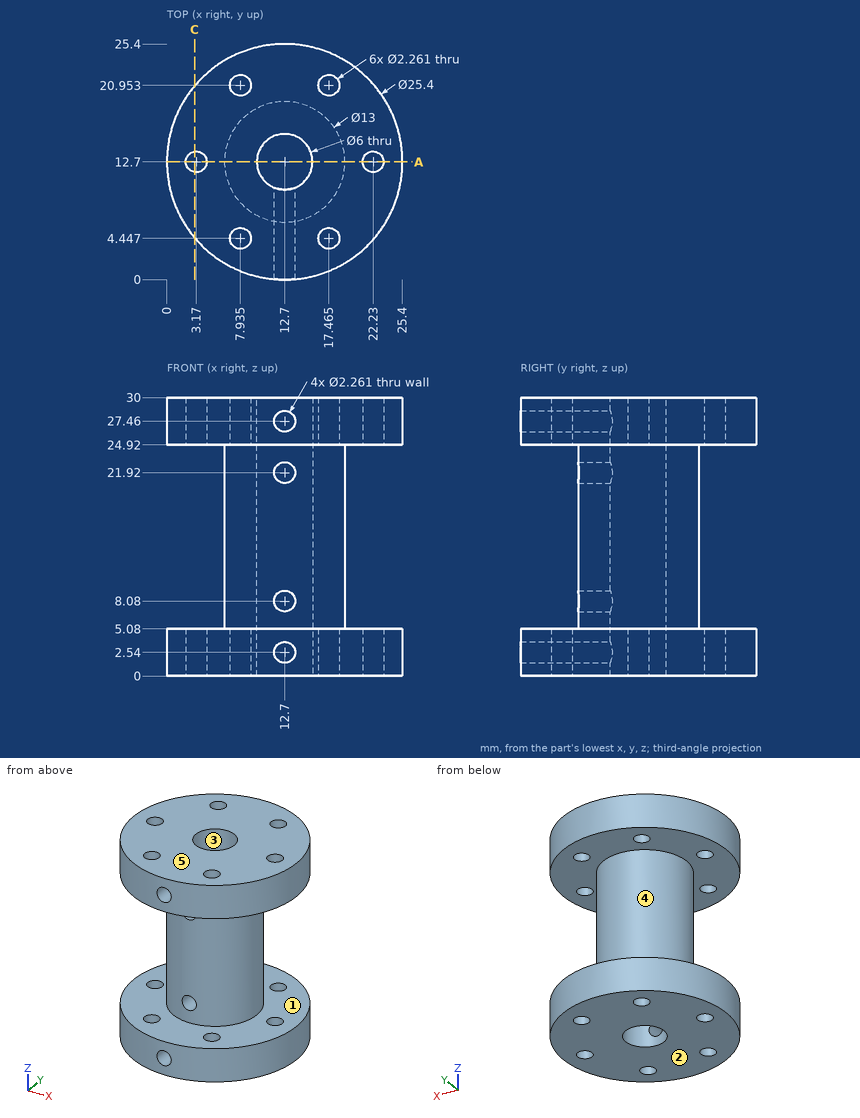
The figure shows three views and two pictorial views of one solid part (mm, origin at its lowest corner). Answer the questions. A direction names the side the tool comes from. Round coordinates to 2 decimals unless told otherwise and drop trailing zeros. Loops run counter-clockwise (first coordinate to the right, second up) from the corner with the lowest first, then second, coordinate; pieces in that order, holes last. Notation, with made-up numbers: (-23, 28) - (11, 28) arc R15 cw to (11, 43) - close; hole circle Ø2 at (32.25, -8.5). An arc over 180 degrees is marked (long way). One line per question, with ' | ' between items. Start each with the question number.
Q1. Flat-ended cylindrical pins translate along their axes: pin 1 (10 mm diameter, centred on x = 19.5, z = 17.5, fed in from -Y); pin 2 (6 mm diameter, centred on x = 9, z = 18, fed in from -Y); pin 3 (5 mm diameter, centred on x = 20, z = 13.5, fed in from -Y). Find the tip coordinate at first contact, or state that the pin passes through.
Q2. Section A-A on y = 12.7 is taken. Count the separate pieces of the cut face and the enclosed holes in it, plus the area to 3 significant figures.
Q3. Section C-C on x = 3 is taken. Give the vertices of the cut face in (y, z), plus the area to 3 significant figures.
Q4. For a pull along X with two mould halves and no side action, classify the marked faces 3, 4 and 5 as +X half, -X half, draft (parallel to the pull), parting line (faces both ways), or undercut.
Q5. For the marked faces 1 and 2, determine the directions among +Z, -Z, +X, -X, +Y, -Y from which every point of the face is accessible in a straight line to the end or side of a thin tool.
Q6. Find the intervals of material crossed by L1, parallel to Z at x = 12.7, y = 7.6; L2, parallel to Z at x = 20.5, y = 12.25; L3, parallel to Y at x = 12.7, z = 7, in increasing order.
Established:
1) pin 1: y = 6.45 | pin 2: y = 6.24 | pin 3: y = 8.32
2) separate pieces: 6 | enclosed holes: 0 | area: 290 mm²
3) outline: (4.5, 0) - (11.58, 0) - (11.58, 5.08) - (4.5, 5.08) - close; (4.5, 24.92) - (11.58, 24.92) - (11.58, 30) - (4.5, 30) - close; (13.82, 0) - (20.9, 0) - (20.9, 5.08) - (13.82, 5.08) - close; (13.82, 24.92) - (20.9, 24.92) - (20.9, 30) - (13.82, 30) - close | area: 144 mm²
4) face 3: undercut | face 4: parting line | face 5: draft
5) face 1: none | face 2: -Z, +X, -X, +Y, -Y
6) L1: 0 to 1.41, 3.67 to 6.95, 9.21 to 20.79, 23.05 to 26.33, 28.59 to 30 | L2: 0 to 5.08, 24.92 to 30 | L3: 15.7 to 19.2
